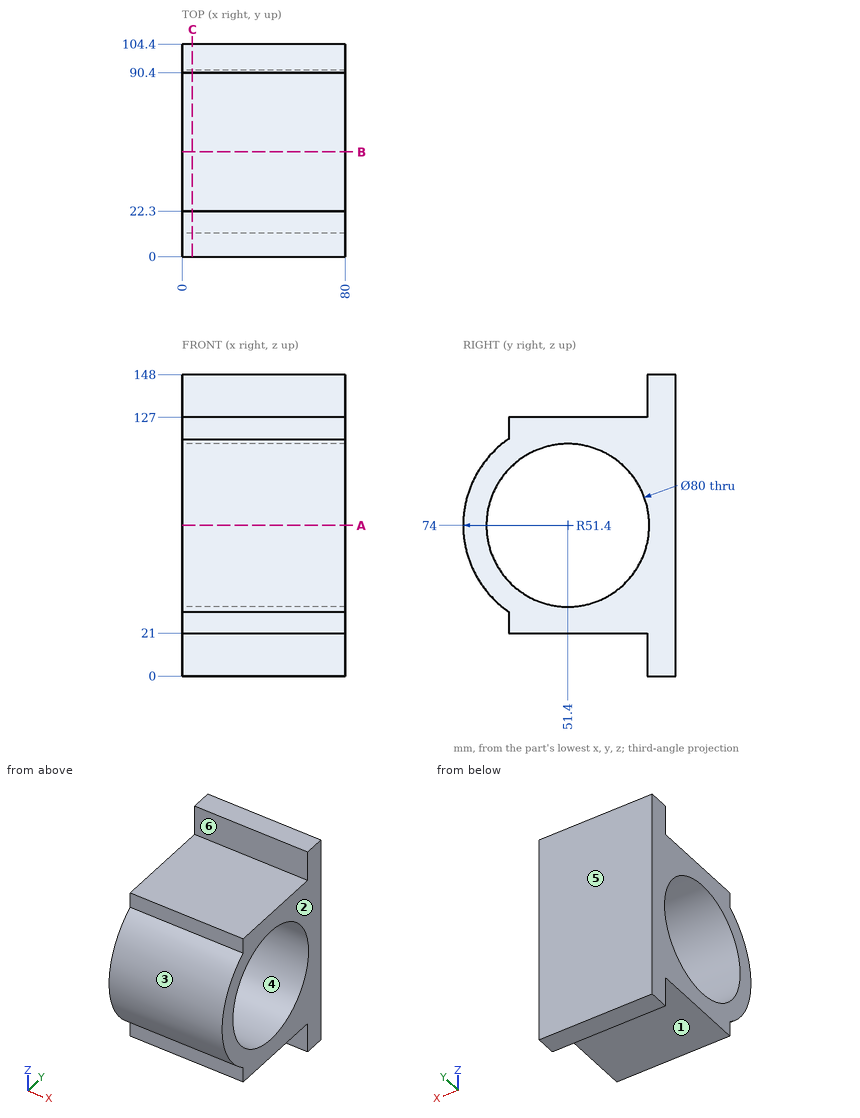
Job drawing, mm, ordinate dimensions from the low corner. One solid piece. A direction names the side the tool comes from. Coordinates: 2 decimals unless noted, no trailing zeros. Write each loop counter-clockwise with the first axis right and the second up, starting at its lowest first coordinate (ties: lowest second). Pieces come first, ordered by that corner, then holes. Notation, with made-up numbers: (15.5, 35.5) - (47.5, 35.5) arc R12 ccw to (47.5, 44.5) - close; hole circle Ø8 at (77, 54.25). An arc over 180 degrees is marked (long way). Use a Markdown table: item, result. Add a question column.
Item 1: Drill centre lines: L1, parallel to Z at x = 61, y = 53; L2, parallel to Y at x = 38.5, z = 74; L3, parallel to Z at x = 47.5, y = 67.5. Where is each one in solid material? Low to high. Write a range as from..to.
Item 2: Band-saw the part on C-C, the plane x = 5. Give the cut face in (y, z).
Item 3: 3-axis set-ups, long thin cutter, end or side, ignore diameter. For the marked faces 5 and 6: which of +Z, -Z, +X, -X, +Y, -Y reach the whole face in a straight line?
Item 4: Band-saw the part on A-A, the plane z = 74. Give the cut face in (x, y), and give its area (3 significant figures).
Item 5: Mould opens along Z. For the marked faces 1, 2, 3 and 4 say: pulls with the +Z half, pulls with the -Z half, needs draft (parallel to the pull), parting line crosses it, or undercut.
Item 6: Band-saw the part on B-B, the plane y = 51.4. Give the cut face in (x, z), and give its area (3 significant figures).
Item 7: Flat gauge pins, fed straight in: pin 1 (1 mm diameter, centred on y = 51, z = 23, fed in from -X); pin 2 (10 mm diameter, centred on x = 62.5, y = 16.5, fed in from -Z); pin 3 (20.5 mm diameter, centred on x = 23, y = 43.5, fed in from +Z); pin 4 (17 mm diameter, centred on x = 43, z = 138, fed in from -Y). Where does each tip first touch, or does it go through?
Numbers:
| question | item | result |
|---|---|---|
| 1 | L1 | 21..34.03, 113.97..127 |
| 1 | L2 | 0..11.4, 91.4..104.4 |
| 1 | L3 | 21..37.38, 110.62..127 |
| 2 | outline | (22.3, 21) - (90.4, 21) - (90.4, 0) - (104.4, 0) - (104.4, 148) - (90.4, 148) - (90.4, 127) - (22.3, 127) - (22.3, 116.37) arc R51.4 ccw to (22.3, 31.63) - close; hole circle Ø80 at (51.4, 74) |
| 3 | face 5 | +Z, -Z, +X, -X, +Y |
| 3 | face 6 | +Z, +X, -X, -Y |
| 4 | outline | (0, 0) - (80, 0) - (80, 11.4) - (0, 11.4) - close; (0, 91.4) - (80, 91.4) - (80, 104.4) - (0, 104.4) - close |
| 4 | area | 1,950 mm2 |
| 5 | face 1 | pulls with the -Z half |
| 5 | face 2 | needs draft |
| 5 | face 3 | parting line crosses it |
| 5 | face 4 | undercut |
| 6 | outline | (0, 21) - (80, 21) - (80, 34) - (0, 34) - close; (0, 114) - (80, 114) - (80, 127) - (0, 127) - close |
| 6 | area | 2,080 mm2 |
| 7 | pin 1 | x = 0 |
| 7 | pin 2 | z = 32.19 |
| 7 | pin 3 | z = 127 |
| 7 | pin 4 | y = 90.4 |
